```python
from build123d import *

# Parameters (mm, degrees)
F0_W     = 108.7436452508
F0_H     = 91.3013890386
F1_DEPTH = 50.8
F2_R     = 25.409051706
F3_DEPTH = 62.484
F4_T     = -2.54
F5_R     = 14.8578389164
F6_DEPTH = 177.8
F7_R     = 14.4786681192
F8_DEPTH = 177.8


with BuildPart() as f1:
    # F0 (on Top) → F1 (new body)
    with BuildSketch(Plane.XY):
        Rectangle(F0_W, F0_H)
    extrude(amount=F1_DEPTH)

    # F2 (on face) → F3 (join)
    with BuildSketch(Plane.XY.offset(50.8)):
        Circle(F2_R)
    extrude(amount=-F3_DEPTH)

    # F4
    f4_openings = [f1.faces().sort_by_distance(p)[0] for p in [
        (0, 0, -11.684),
    ]]
    offset(amount=F4_T, openings=f4_openings, kind=Kind.INTERSECTION)

    # F5 (on face) → F6 (join)
    with BuildSketch(Plane.YZ.offset(54.3718226254)):
        with Locations((0, 24.9464344233)):
            Circle(F5_R)
    extrude(amount=F6_DEPTH)

    # F7 (on face) → F8 (join)
    with BuildSketch(Plane(origin=(0, 45.6506945193, 0), x_dir=(-1, 0, 0), z_dir=(0, 1, 0))):
        with Locations((0, 28.3211600035)):
            Circle(F7_R)
    extrude(amount=F8_DEPTH)


solid = f1.part
```
Here's how the part is built. I have some questions about the finished solid (model axes, mm). A direction names the side the tool comes from. Give positions to 0.01 mm unless a question says otherwise; leave off trailing zeros. Loops run counter-clockwise (first coordinate to the right, second up) from the corner with the lowest first, then second, coordinate; pieces in that order, holes last. Notation, with made-up numbers: M 68.25,-23 L 124.25,-23 A15 cw 124.25,-15 Z; hole C -16.5,-10.75 d6. An arc over 180 degrees is marked long. Use one line per item in the form item = value. Start each with the question number.
Q1. I need wall thicknesses on line 1 along Y through (x, z) = (0, -3.25); line 2 along Z through (x, y) = (23.5, 41.5); line 3 along Y through (x, z) = (-15, 35.5). Which ranges of each line are inside material? Lowest first, please.
Q2. Thinking about a two-plate mould opening in X: for faces 4 (the cylindrical face through (3.139, 133.306, 14.187)), 5 (the flat face through (-51.832, -1, 25)), 6 (the cylindrical face through (142.03, -3.22, 10.44)), which applies, +X half, -X half, draft (parallel to the pull), parting line (faces both ways), or undercut?
Q3. If we section it at D-D (z = -3.5): Write out the boundary of the cut face in (x, y), then the cut area to 3 significant figures.
Q4. If we section it at B-B (y = 0): Write out the boundary of the cut face in (x, z).
Q5. Which directions (+Z, -Z, +X, -X, +Y, -Y) give clear straight access to the entire face, cutting with the end or side of a thin tool? Please do faces 1 (the flat face through (-12, 20, 2.54)), 2 (the cylindrical face through (-18.148, -13.915, -4.472)), 3 (the flat face through (-54.372, -1, 25)).
Q6. Will these pins go through, and if not, where does the flat tip stop? pin 1 Ø10 at (x, y) = (33.5, 43.5) entering from -Z; pin 2 Ø3 at (y, z) = (59.5, 25) entering from +X; pin 3 Ø12 at (x, z) = (86.5, 40.5) entering from -Y.
Q7. If we section it at C-C (z = 34.5): Write out the boundary of the cut face in (x, y).
Q8. If we section it at A-A (x = 0): Write out the boundary of the cut face in (y, z), then the cut area to 3 significant figures.
Taken from the geometry:
q1.line_1 = -25.41 to -22.87, 22.87 to 25.41
q1.line_2 = 0 to 2.54, 48.26 to 50.8
q1.line_3 = -45.65 to -43.11, 43.11 to 45.65
q2.face_4 = parting line
q2.face_5 = undercut
q2.face_6 = draft
q3.outline = C 0,0 d50.82; hole C 0,0 d45.74
q3.area = 385 mm^2
q4.outline = M -54.37,0 L -25.41,0 L -25.41,-11.68 L -22.87,-11.68 L -22.87,2.54 L -51.83,2.54 L -51.83,48.26 L 51.83,48.26 L 51.83,2.54 L 22.87,2.54 L 22.87,-11.68 L 25.41,-11.68 L 25.41,0 L 54.37,0 L 54.37,10.09 L 232.17,10.09 L 232.17,39.8 L 54.37,39.8 L 54.37,50.8 L -54.37,50.8 Z
q5.face_1 = none
q5.face_2 = -Z
q5.face_3 = +Z, -Z, -X, +Y, -Y
q6.pin_1 = 0
q6.pin_2 = 14.36
q6.pin_3 = -11.38
q7.outline = M -54.37,-45.65 L 54.37,-45.65 L 54.37,-11.38 L 232.17,-11.38 L 232.17,11.38 L 54.37,11.38 L 54.37,45.65 L 13.09,45.65 L 13.09,223.45 L -13.09,223.45 L -13.09,45.65 L -54.37,45.65 Z; hole M -51.83,-43.11 L 51.83,-43.11 L 51.83,43.11 L -51.83,43.11 Z
q8.outline = M -45.65,0 L -25.41,0 L -25.41,-11.68 L -22.87,-11.68 L -22.87,2.54 L -43.11,2.54 L -43.11,48.26 L 43.11,48.26 L 43.11,2.54 L 22.87,2.54 L 22.87,-11.68 L 25.41,-11.68 L 25.41,0 L 45.65,0 L 45.65,13.84 L 223.45,13.84 L 223.45,42.8 L 45.65,42.8 L 45.65,50.8 L -45.65,50.8 Z
q8.area = 5,790 mm^2
